Input: dimensioned drawing with shaded views. Units: mm. Origin: part minimum x, y, z. A direction names the side the tool comes from. Give positions to 0.01 mm unless a question says otherwise; leave off trailing zeros. Write each loop counter-clockwise with the first axis right and the second up, starting at its lowest first coordinate (ties: lowest second). Pieces come first, ordered by that corner, then holes. Notation, with made-up numbers: (88.5, 74) -> (129.5, 74) arc R30 cw to (129.5, 107) -> close; hole circle Ø7 at (21.25, -4.75). An arc over 180 degrees is marked (long way). Answer as a JSON object with one key per item and string values.
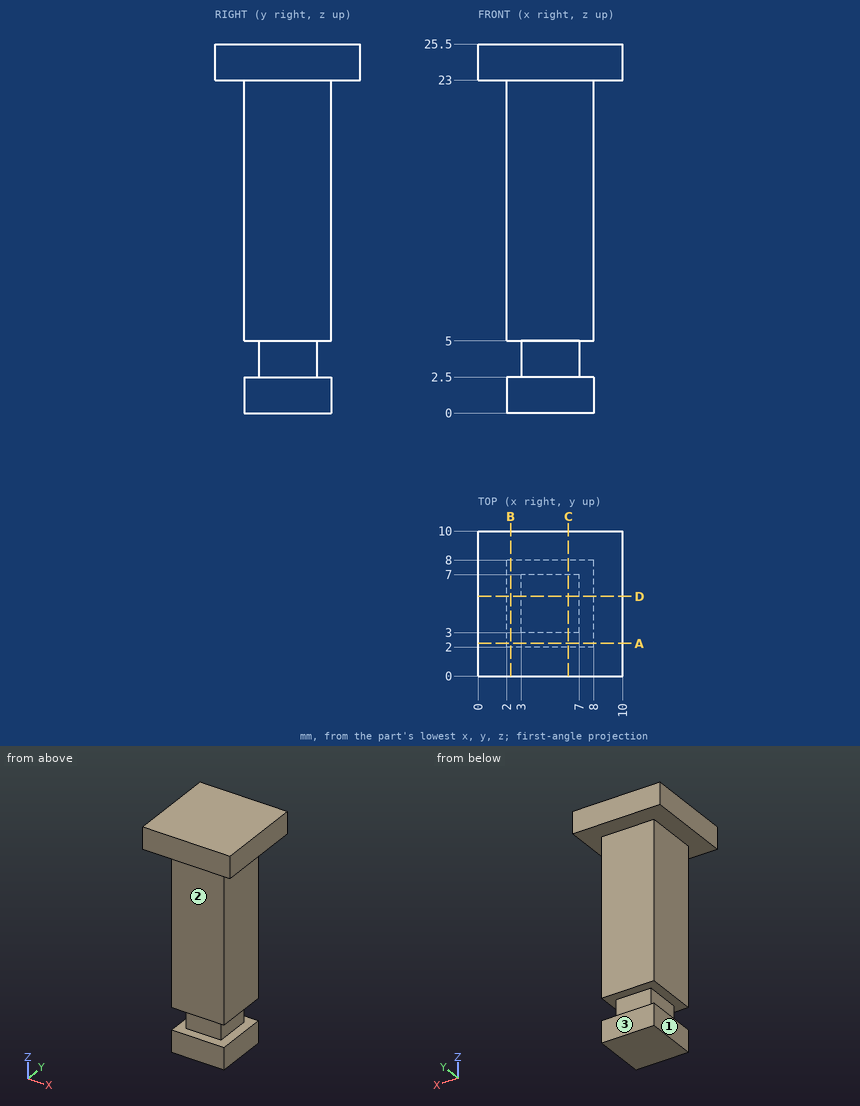
Q1. Cut plane C-C (x = 6.25). Return the cut outline in (y, z).
Values:
{"outline": "(0, 23) -> (2, 23) -> (2, 5) -> (3, 5) -> (3, 2.5) -> (2, 2.5) -> (2, 0) -> (8, 0) -> (8, 2.5) -> (7, 2.5) -> (7, 5) -> (8, 5) -> (8, 23) -> (10, 23) -> (10, 25.5) -> (0, 25.5) -> close"}
Q2. Set-up query: the marked faces 1, 2 and 3. Return all of +Z, -Z, +X, -X, +Y, -Y with unobstructed straight access to the full face (end or side cutting, diameter ignored); none if empty.
Values:
{"face 1": "-Z, -X, +Y, -Y", "face 2": "-Z, +X, -X, -Y", "face 3": "-Z, +X, -X, +Y"}
Q3. Material intervals for L1, parallel to Z at x = 6.5, y = 2.75; L2, parallel to X at y = 4.5, z = 13.5, sorted ascending. Write a range as from..to.
Values:
{"L1": "0..2.5, 5..25.5", "L2": "2..8"}
Q4. First-contact query: P1, Ø2, axis at y = 4, z = 1.5, coming from the -X side; P2, Ø3, axis at x = 6, z = 2, coming from the +Y side; P3, Ø3, axis at y = 5.5, z = 0.5, coming from the +X side. Flat tips, straight axial feed; report the tip coordinate or a pass-through.
Values:
{"P1": "x = 2", "P2": "y = 8", "P3": "x = 8"}
Q5. Cut plane A-A (y = 2.25). Return the cut outline in (x, z).
Values:
{"outline": "(0, 23) -> (2, 23) -> (2, 5) -> (8, 5) -> (8, 23) -> (10, 23) -> (10, 25.5) -> (0, 25.5) -> close; (2, 0) -> (8, 0) -> (8, 2.5) -> (2, 2.5) -> close"}
